Can you work these out from the drawing? Everything is in mm from the part's minimum corner. A direction names the side the tool comes from. Coordinates: 2 decimals unless noted, no trailing zeros. Loops run counter-clockwise (first coordinate to the right, second up) from the corner with the lowest first, then second, coordinate; pieces in that order, holes last. Notation, with made-up numbers: (-27, 79.5) -> (-14, 79.5) arc R23 ccw to (-14, 116.5) -> close; hole circle Ø4 at (-23, -17). An arc over 180 degrees is marked (long way). Put each result on its own line as item: value. Start each with the question number.
Item 1: If we section it at C-C on z = 46.5: Please give me the cut outline in (x, y).
Item 2: We'd pull the mould along X, two halves only. Please class the marked faces 3, 4 and 5: pulls with the +X half, pulls with the -X half, needs draft (parallel to the pull), parting line crosses it, or undercut.
Item 3: For the marked faces 1 and 2, which set-ups out of +Z, -Z, +X, -X, +Y, -Y let a thin tool reach every point of the face, with its end or its side?
Item 4: If we section it at B-B on x = 31: Please give me the cut outline in (y, z).
Item 5: Will this pin go through, and if not, where does the flat tip stop? P1, Ø12, axis at x = 92, z = 57, coming from the -Y side.
Item 6: Please list where these lines run through material, in increasing order: L1, parallel to X at y = 22, z = 68; L2, parallel to Z at x = 201, y = 36.5; L3, parallel to Y at x = 195, z = 96.5. Write a range as from..to.
Item 7: If we section it at A-A on y = 16.5: Please give me the cut outline in (x, z).
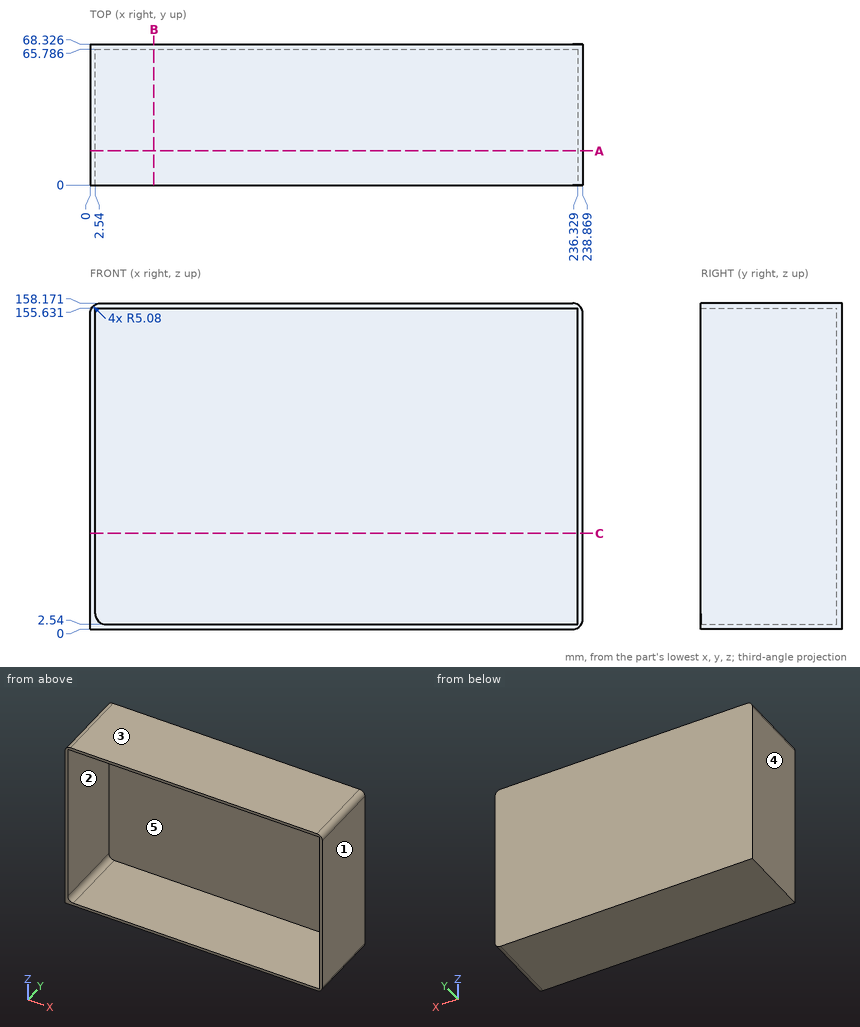
Solutions:
1. outline: (0, 0) -> (2.54, 0) -> (2.54, 65.79) -> (236.33, 65.79) -> (236.33, 0) -> (238.87, 0) -> (238.87, 68.33) -> (0, 68.33) -> close
2. face 3: needs draft
2. face 4: pulls with the -X half
2. face 5: undercut
3. face 1: +Z, -Z, +X, +Y, -Y
3. face 2: -Y
4. outline: (0, 0) -> (68.33, 0) -> (68.33, 158.17) -> (0, 158.17) -> (0, 155.63) -> (65.79, 155.63) -> (65.79, 2.54) -> (0, 2.54) -> close
5. P1: y = 65.79
6. L1: 0..2.54, 236.33..238.87
6. L2: 0..2.54, 155.63..158.17
6. L3: 65.79..68.33
7. outline: (0, 0) -> (233.79, 0) arc R5.08 ccw to (238.87, 5.08) -> (238.87, 153.09) arc R5.08 ccw to (233.79, 158.17) -> (5.08, 158.17) arc R5.08 ccw to (0, 153.09) -> close; hole (2.54, 7.62) arc R5.08 ccw to (7.62, 2.54) -> (236.33, 2.54) -> (236.33, 155.63) -> (2.54, 155.63) -> close
